The model under review builds one solid part; all positions refer to its coordinate system, in mm. Face numbers are marked on the shaded views. Give positions to 0.01 mm unless a question says otherwise; leave off trailing zeros. Loops run counter-clockwise (first coordinate to the right, second up) from the corner with the lowest first, then second, coordinate; pieces in that order, holes last. Notation, with made-up numbers: M -30,87 L -10,87 A27 ccw -10,125 Z; hole C 29.5,68.5 d8. An arc over 180 degrees is marked long. Return JSON: item names as keys, results as strings.
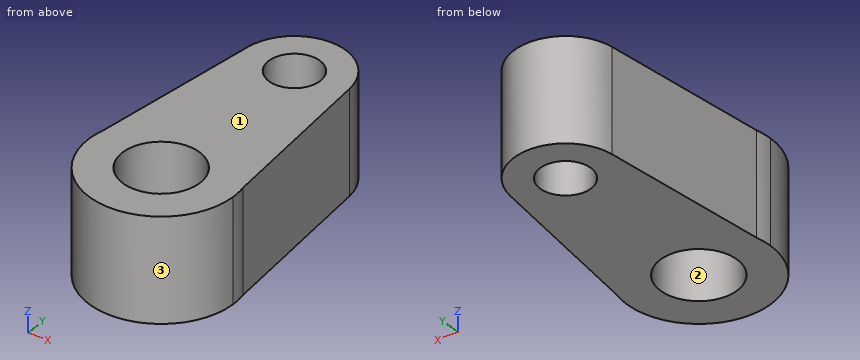
```python
from build123d import *

# Parameters (mm, degrees)
F0_R     = 47.385597
F0_R_2   = 31.425438
F1_DEPTH = 127


with BuildPart() as f1:
    # F0 (on Top) → F1 (new body)
    with BuildSketch(Plane.XY):
        with BuildLine():
            Line((-86.634222, 19.942958), (-88.9, 0))
            ThreePointArc((-88.9, 0), (0, -88.9), (88.9, 0))
            Line((88.9, 0), (86.634222, 19.942958))
            ThreePointArc((86.634222, 19.942958), (0, 88.9), (-86.634222, 19.942958))
        make_face()
        Circle(F0_R, mode=Mode.SUBTRACT)
        with BuildLine():
            ThreePointArc((-86.634222, 19.942958), (-88.331739, 10.035628), (-88.9, 0))
            Line((-88.9, 0), (-86.634222, 19.942958))
        make_face()
        with BuildLine():
            Line((86.634222, 19.942958), (88.9, 0))
            ThreePointArc((88.9, 0), (88.331739, 10.035628), (86.634222, 19.942958))
        make_face()
        with BuildLine():
            Line((-63.0941, 227.138758), (-86.634222, 19.942958))
            ThreePointArc((-86.634222, 19.942958), (0, 88.9), (86.634222, 19.942958))
            Line((86.634222, 19.942958), (63.0941, 227.138758))
            ThreePointArc((63.0941, 227.138758), (63.398444, 223.560347), (63.5, 219.970453))
            ThreePointArc((63.5, 219.970453), (-3.589894, 156.572009), (-63.0941, 227.138758))
        make_face()
        with BuildLine():
            ThreePointArc((63.0941, 227.138758), (0, 283.470453), (-63.0941, 227.138758))
            ThreePointArc((-63.0941, 227.138758), (-3.589894, 156.572009), (63.5, 219.970453))
            ThreePointArc((63.5, 219.970453), (63.398444, 223.560347), (63.0941, 227.138758))
        make_face()
        with Locations((0, 219.970453)):
            Circle(F0_R_2, mode=Mode.SUBTRACT)
    extrude(amount=F1_DEPTH)


solid = f1.part
```
1) Consider section B-B on y = -21.5. Write out the cut boundary in (x, z).
From the geometry:
{"outline": "M -86.26,0 L -42.23,0 L -42.23,127 L -86.26,127 Z; M 42.23,0 L 86.26,0 L 86.26,127 L 42.23,127 Z"}
2) Consider section A-A on x = 0. Write out the cut boundary in (y, z), then the cut area to 3 significant figures.
From the geometry:
{"outline": "M -88.9,0 L -47.39,0 L -47.39,127 L -88.9,127 Z; M 47.39,0 L 188.55,0 L 188.55,127 L 47.39,127 Z; M 251.4,0 L 283.47,0 L 283.47,127 L 251.4,127 Z", "area": "27,300 mm²"}
3) Consider section C-C on z = 104. Write out the cut boundary in (x, y), then the cut area to 3 significant figures.
From the geometry:
{"outline": "M -88.9,0 A88.9 ccw 88.9,0 A88.9 ccw 86.63,19.94 L 63.09,227.14 A63.5 ccw -63.09,227.14 L -86.63,19.94 A88.9 ccw Z; hole C 0,0 d94.77; hole C 0,219.97 d62.85", "area": "42,200 mm²"}
4) Consider section D-D on y = 145.5. Write out the cut boundary in (x, z).
From the geometry:
{"outline": "M -72.37,0 L 72.37,0 L 72.37,127 L -72.37,127 Z"}
5) Wall thickness on L1, parallel to Y at x = -1.5, z = 51; L2, parallel to Y at x = -4, z = 66; L3, parallel to Y at x = 32, z = 65: over which ranges is each line inside the solid? List them lowest first. Write a range as from..to.
From the geometry:
{"L1": "-88.89..-47.36, 47.36..188.58, 251.36..283.45", "L2": "-88.81..-47.22, 47.22..188.8, 251.14..283.34", "L3": "-82.94..-34.95, 34.95..274.82"}
6) Insertion check: pin 1 (8 mm diameter, centred on x = -52, z = 68.5, fed in from +Y); pin 2 (1 mm diameter, centred on x = -40.5, z = 71.5, fed in from -Y); pin 3 (4 mm diameter, centred on x = -49.5, z = 57, fed in from -Y). Each pin has a flat end and moves straight along its axis. Give the tip position at first contact, or say it passes through.
From the geometry:
{"pin 1": "y = 261.54", "pin 2": "y = -79.39", "pin 3": "y = -75.15"}
7) The part is to be moulded in two halves that separate along X. For the marked faces 1, 2 and 3, say which applies: released by +X, released by -X, zero draft, split by the parting line, or undercut.
From the geometry:
{"face 1": "zero draft", "face 2": "undercut", "face 3": "split by the parting line"}
